CAD build for the part. Positions are in the model's coordinates, mm. Coordinates: 2 decimals unless noted, no trailing zeros. Loops run counter-clockwise (first coordinate to the right, second up) from the corner with the lowest first, then second, coordinate; pieces in that order, holes last. Notation, with made-up numbers: (76.25, 26.25) -> (115.25, 26.25) arc R15 ccw to (115.25, 52.25) -> close; hole circle Ø3 at (68.25, 75). An arc over 180 degrees is marked (long way). Write each question's results on one line, items separated by ' | '.
from build123d import *

# Parameters (mm, degrees)
SKETCH1_W               = 27
SKETCH1_H               = 50
BOSS_EXTRUDE1_DEPTH     = 1.5
SKETCH2_W               = 12
SKETCH2_H               = 3
BOSS_EXTRUDE2_DEPTH     = 1.5
SKETCH4_W               = 3
SKETCH4_H               = 25
CUT_EXTRUDE1_DEPTH      = 2.5
CUT_EXTRUDE1_DEPTH_BACK = 2.5
FILLET1_R               = 3
SKETCH5_W               = 6
SKETCH5_H               = 3
CUT_EXTRUDE2_DEPTH      = 2.5
CUT_EXTRUDE2_DEPTH_BACK = 2.5


with BuildPart() as part:
    # Sketch1 → Boss-Extrude1 (new body, symmetric)
    with BuildSketch(Plane(origin=(0, 0, 0), x_dir=(1, 0, 0), z_dir=(0, 1, 0))):
        Rectangle(SKETCH1_W, SKETCH1_H)
    extrude(amount=BOSS_EXTRUDE1_DEPTH, both=True)

    # Sketch2 → Boss-Extrude2 (add, symmetric)
    with BuildSketch(Plane(origin=(0, 0, 0), x_dir=(1, 0, 0), z_dir=(0, 1, 0))):
        with Locations((0, -26.5)):
            Rectangle(SKETCH2_W, SKETCH2_H)
    extrude(amount=BOSS_EXTRUDE2_DEPTH, both=True)

    # Sketch4 → Cut-Extrude1 (cut, two sides)
    with BuildSketch(Plane(origin=(0, 0, 0), x_dir=(1, 0, 0), z_dir=(0, 1, 0))) as cut_extrude1_sk:
        with Locations((-9, -7.5)):
            Rectangle(SKETCH4_W, SKETCH4_H)
        with Locations((9, -7.5)):
            Rectangle(SKETCH4_W, SKETCH4_H)
    extrude(amount=CUT_EXTRUDE1_DEPTH, mode=Mode.SUBTRACT)
    extrude(cut_extrude1_sk.sketch, amount=-CUT_EXTRUDE1_DEPTH_BACK, mode=Mode.SUBTRACT)

    # Fillet1
    fillet1_edges = [part.edges().sort_by_distance(p)[0] for p in [
        (-13.5, 0, -25),
        (13.5, 0, -25),
    ]]
    fillet(fillet1_edges, radius=FILLET1_R)

    # Sketch5 → Cut-Extrude2 (cut, two sides)
    with BuildSketch(Plane(origin=(0, 0, 0), x_dir=(1, 0, 0), z_dir=(0, 1, 0))) as cut_extrude2_sk:
        with Locations((0, 23.5)):
            Rectangle(SKETCH5_W, SKETCH5_H)
    extrude(amount=CUT_EXTRUDE2_DEPTH, mode=Mode.SUBTRACT)
    extrude(cut_extrude2_sk.sketch, amount=-CUT_EXTRUDE2_DEPTH_BACK, mode=Mode.SUBTRACT)


solid = part.part
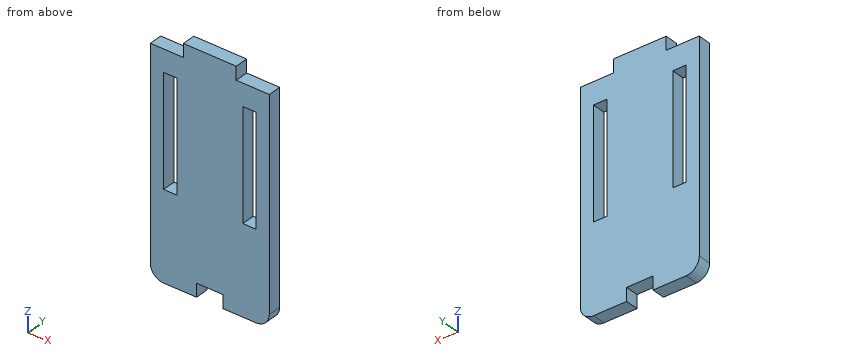
1) Slice it at C-C (z = -4.5). Write the cut outline in (x, y).
Outcome:
outline: (-13.5, -1.5) -> (-10.5, -1.5) -> (-10.5, 1.5) -> (-13.5, 1.5) -> close; (-7.5, -1.5) -> (7.5, -1.5) -> (7.5, 1.5) -> (-7.5, 1.5) -> close; (10.5, -1.5) -> (13.5, -1.5) -> (13.5, 1.5) -> (10.5, 1.5) -> close
2) Drill centre lines: L1, parallel to X at y = -0.35, z = 2.5; L2, parallel to Z at x = 7.75, y = -0.35; L3, parallel to Z at x = 1, y = -0.4. Where is each one in solid material? Low to high. Write a range as from..to.
Outcome:
L1: x = -13.5..-10.5, -7.5..7.5, 10.5..13.5 | L2: z = -25..-5, 20..25 | L3: z = -22..28
3) Pin check, flat tips, straight feed: pin 1 (1.5 mm diameter, centred on y = 0.5, z = -24, fed in from +X); pin 2 (1.5 mm diameter, centred on x = 8.5, y = 0, fed in from +Z); pin 3 (0.9 mm diameter, centred on x = -1, y = 0, fed in from -Z). Stop position of each tip, or through.
Outcome:
pin 1: stops at x = 13.23 | pin 2: stops at z = 25 | pin 3: stops at z = -22
4) Slice it at D-D (x = -0.75). Write the cut outline in (y, z).
Outcome:
outline: (-1.5, -22) -> (1.5, -22) -> (1.5, 28) -> (-1.5, 28) -> close
5) Slice it at B-B (y = 0.15). Write the cut outline in (x, z), then the cut area to 3 significant figures.
Outcome:
outline: (-13.5, -22) arc R3 ccw to (-10.5, -25) -> (-3, -25) -> (-3, -22) -> (3, -22) -> (3, -25) -> (10.5, -25) arc R3 ccw to (13.5, -22) -> (13.5, 25) -> (6, 25) -> (6, 28) -> (-6, 28) -> (-6, 25) -> (-13.5, 25) -> close; hole (-10.5, -5) -> (-7.5, -5) -> (-7.5, 20) -> (-10.5, 20) -> close; hole (7.5, -5) -> (10.5, -5) -> (10.5, 20) -> (7.5, 20) -> close | area: 1,210 mm^2
6) Slice it at A-A (x = -9.25). Write the cut outline in (y, z).
Outcome:
outline: (-1.5, -25) -> (1.5, -25) -> (1.5, -5) -> (-1.5, -5) -> close; (-1.5, 20) -> (1.5, 20) -> (1.5, 25) -> (-1.5, 25) -> close
